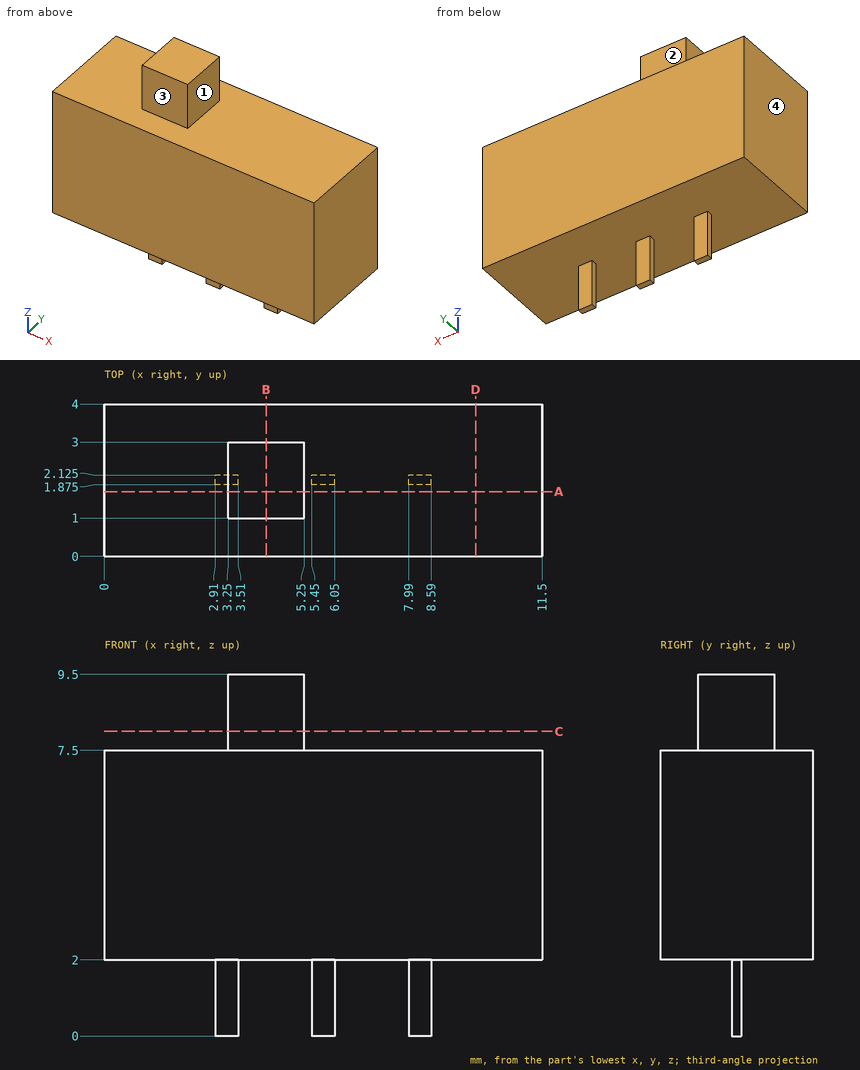
Source: three-view drawing plus pictorial views. Frame: mm from the lowest corner of the part. A direction names the side the tool comes from. Round coordinates to 2 decimals unless told otherwise and drop trailing zeros. Loops run counter-clockwise (first coordinate to the right, second up) from the corner with the lowest first, then second, coordinate; pieces in that order, holes last.
Q1. Section D-D on x = 9.75. Return loops of the section in (y, z).
Q2. Access query for the marked faces 1, 2, 3 and 4. Directions: +Z, -Z, +X, -X, +Y, -Y. A direction counts if a zero-diameter tool reaches every point of the face in a straight line with its end or side. Return the directions, or none.
Q3. Material intervals for L1, parallel to Z at x = 2.25, y = 2.6; L2, parallel to X at y = 2.55, z = 8.75; L3, parallel to Y at x = 4.5, z = 9, sorted ascending.
Q4. Section A-A on y = 1.7. Return loops of the section in (x, z).
Q5. Pin query (flat end, axial travel): P1, Ø2, axis at x = 8, y = 1, coming from the +Z side; P2, Ø1.5, axis at x = 9.5, z = 1, coming from the -Y side; P3, Ø0.5, axis at x = 8, z = 0.5, coming from the +Y side (3 decimals); P4, Ø0.6, axis at x = 4.5, z = 8, coming from the +Y side. Return the tip coordinate at first contact, or that it passes through.
Q6. Section B-B on x = 4.25. Return loops of the section in (y, z).
Q7. Section C-C on z = 8. Return loops of the section in (x, y).
Evaluation:
1. outline: (0, 2) - (4, 2) - (4, 7.5) - (0, 7.5) - close
2. face 1: +Z, +X, +Y, -Y
2. face 2: +Z, +X, -X, +Y
2. face 3: +Z, +X, -X, -Y
2. face 4: +Z, -Z, -X, +Y, -Y
3. L1: z = 2 to 7.5
3. L2: x = 3.25 to 5.25
3. L3: y = 1 to 3
4. outline: (0, 2) - (11.5, 2) - (11.5, 7.5) - (5.25, 7.5) - (5.25, 9.5) - (3.25, 9.5) - (3.25, 7.5) - (0, 7.5) - close
5. P1: stops at z = 7.5
5. P2: passes through
5. P3: stops at y = 2.125
5. P4: stops at y = 3
6. outline: (0, 2) - (4, 2) - (4, 7.5) - (3, 7.5) - (3, 9.5) - (1, 9.5) - (1, 7.5) - (0, 7.5) - close
7. outline: (3.25, 1) - (5.25, 1) - (5.25, 3) - (3.25, 3) - close
